Model file for the job. Use its own axes, mm. Round coordinates to 2 decimals unless told otherwise and drop trailing zeros. Loops run counter-clockwise (first coordinate to the right, second up) from the corner with the lowest first, then second, coordinate; pieces in that order, holes last. Notation, with made-up numbers: (34.25, 78.25) -> (46.25, 78.25) arc R5 cw to (46.25, 84.25) -> close; hole circle Ø10 at (27, 11). An arc over 180 degrees is marked (long way). Use a Markdown table: item, result.
from build123d import *

# Parameters (mm, degrees)
SKETCH1_W                                           = 63
SKETCH1_H                                           = 38
BOSS_EXTRUDE1_DEPTH                                 = 5
CBORE_FOR_2_BINDING_HEAD_MACHINE_SCREW2_D           = 2.4384
CBORE_FOR_2_BINDING_HEAD_MACHINE_SCREW2_CBORE_D     = 5.55752
CBORE_FOR_2_BINDING_HEAD_MACHINE_SCREW2_CBORE_DEPTH = 1.27
CBORE_FOR_2_BINDING_HEAD_MACHINE_SCREW3_D           = 2.4384
CBORE_FOR_2_BINDING_HEAD_MACHINE_SCREW3_CBORE_D     = 5.55752
CBORE_FOR_2_BINDING_HEAD_MACHINE_SCREW3_CBORE_DEPTH = 1.27
CUT_EXTRUDE1_DEPTH                                  = 10
F_2_56_TAPPED_HOLE2_D                               = 1.778
F_2_56_TAPPED_HOLE2_DEPTH                           = 2.46583491
F_2_56_TAPPED_HOLE2_TIP                             = 0.53416509
F_2_56_TAPPED_HOLE3_D                               = 1.778
F_2_56_TAPPED_HOLE3_DEPTH                           = 7.46583491
F_2_56_TAPPED_HOLE3_TIP                             = 0.53416509


with BuildPart() as part:
    # Sketch1 → Boss-Extrude1 (new body)
    with BuildSketch(Plane(origin=(0, 0, 0), x_dir=(1, 0, 0), z_dir=(0, 1, 0))):
        Rectangle(SKETCH1_W, SKETCH1_H)
    extrude(amount=BOSS_EXTRUDE1_DEPTH)

    # CBORE for #2 Binding Head Machine Screw2 (through all)
    with Locations(Plane(origin=(0, 0, 0), x_dir=(-1, 0, 0), z_dir=(0, -1, 0))):
        with Locations((-29, 2.5)):
            CounterBoreHole(CBORE_FOR_2_BINDING_HEAD_MACHINE_SCREW2_D / 2, CBORE_FOR_2_BINDING_HEAD_MACHINE_SCREW2_CBORE_D / 2, CBORE_FOR_2_BINDING_HEAD_MACHINE_SCREW2_CBORE_DEPTH)

    # CBORE for #2 Binding Head Machine Screw3 (through all)
    with Locations(Plane(origin=(0, 0, 0), x_dir=(-1, 0, 0), z_dir=(0, -1, 0))):
        with Locations((-12, -16.5), (17, -16.5)):
            CounterBoreHole(CBORE_FOR_2_BINDING_HEAD_MACHINE_SCREW3_D / 2, CBORE_FOR_2_BINDING_HEAD_MACHINE_SCREW3_CBORE_D / 2, CBORE_FOR_2_BINDING_HEAD_MACHINE_SCREW3_CBORE_DEPTH)

    # Sketch17 → Cut-Extrude1 (cut)
    with BuildSketch(Plane.XZ):
        with BuildLine():
            ThreePointArc((15.55, -2.5), (14.949568901, -1.050431099), (13.5, -0.45))
            Line((13.5, -0.45), (13.5, -2.5))
            Line((13.5, -2.5), (13.5, -4.55))
            ThreePointArc((13.5, -4.55), (14.949568901, -3.949568901), (15.55, -2.5))
        make_face()
        with BuildLine():
            Line((13.5, -2.5), (13.5, -0.45))
            ThreePointArc((13.5, -0.45), (11.45, -2.5), (13.5, -4.55))
            Line((13.5, -4.55), (13.5, -2.5))
        make_face()
    extrude(amount=-CUT_EXTRUDE1_DEPTH, mode=Mode.SUBTRACT)

    # #2-56 Tapped Hole2
    with Locations(Plane(origin=(0, 0, 0), x_dir=(-1, 0, 0), z_dir=(0, -1, 0))):
        with Locations((-13.5, 8.6), (-13.5, -3.6)):
            Hole(F_2_56_TAPPED_HOLE2_D / 2, depth=F_2_56_TAPPED_HOLE2_DEPTH)
            with Locations((0, 0, -(F_2_56_TAPPED_HOLE2_DEPTH + F_2_56_TAPPED_HOLE2_TIP / 2))):  # 118° drill point
                Cone(0, F_2_56_TAPPED_HOLE2_D / 2, F_2_56_TAPPED_HOLE2_TIP, mode=Mode.SUBTRACT)

    # #2-56 Tapped Hole3
    with Locations(Plane(origin=(0, 0, -19), x_dir=(-1, 0, 0), z_dir=(0, 0, -1))):
        with Locations((-12, 2.5), (17, 2.5)):
            Hole(F_2_56_TAPPED_HOLE3_D / 2, depth=F_2_56_TAPPED_HOLE3_DEPTH)
            with Locations((0, 0, -(F_2_56_TAPPED_HOLE3_DEPTH + F_2_56_TAPPED_HOLE3_TIP / 2))):  # 118° drill point
                Cone(0, F_2_56_TAPPED_HOLE3_D / 2, F_2_56_TAPPED_HOLE3_TIP, mode=Mode.SUBTRACT)


solid = part.part
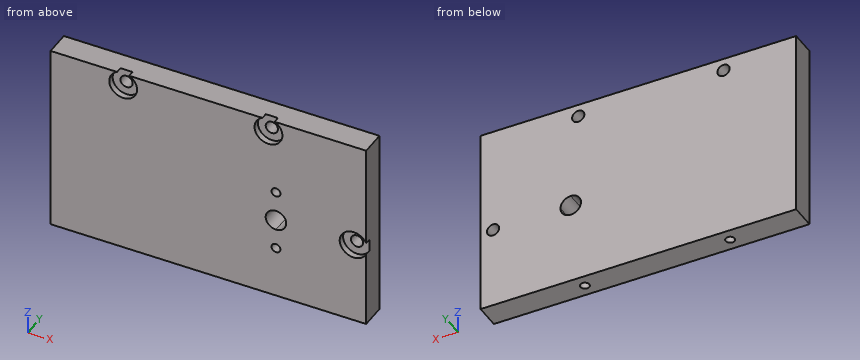
Q1. Drill centre lines: L1, parallel to X at y = 2.35, z = 16.5; L2, parallel to X at y = 0.4, z = -2.5; L3, parallel to X at y = 2.5, z = -15.5. Where is each one in solid material? Low to high. Write a range as from..to.
Results list:
| item | result |
|---|---|
| L1 | x = -31.5..-18.22, -15.78..10.78, 13.22..31.5 |
| L2 | x = -31.5..11.45, 15.55..26.22 |
| L3 | x = -31.5..-17.89, -16.11..11.11, 12.89..31.5 |
Q2. Band-saw the part on A-A, the plane z = 16.5. Give the cut face in (x, y), plus the area to 3 significant figures.
Results list:
| item | result |
|---|---|
| outline | (-31.5, 0) -> (-19.78, 0) -> (-19.78, 1.27) -> (-18.22, 1.27) -> (-18.22, 5) -> (-31.5, 5) -> close; (-15.78, 1.27) -> (-14.22, 1.27) -> (-14.22, 0) -> (9.22, 0) -> (9.22, 1.27) -> (10.78, 1.27) -> (10.78, 5) -> (-15.78, 5) -> close; (13.22, 1.27) -> (14.78, 1.27) -> (14.78, 0) -> (31.5, 0) -> (31.5, 5) -> (13.22, 5) -> close |
| area | 283 mm² |
Q3. Flat gauge pin, fed straight in: pin 1 (3.5 mm diameter, centred on x = 12, z = 16.5, fed in from -Y). Where does the tip first touch, or does it go through?
Results list:
| item | result |
|---|---|
| pin 1 | stops at y = 1.27 |
